Source: three-view drawing plus pictorial views. Frame: mm from the lowest corner of the part. A direction names the side the tool comes from. Round coordinates to 2 decimals unless told otherwise and drop trailing zeros. Order: outer loops, then holes, each group sorted by start corner. A loop starts at its lowest first (then second) coordinate and runs counter-clockwise, first axis right, second up. Notation, with made-up numbers: (-2.5, -20) -> (51.5, -20) arc R19 ccw to (51.5, -16) -> close; hole circle Ø10 at (89, -29). An arc over 180 degrees is marked (long way). Use a Markdown table: item, result.
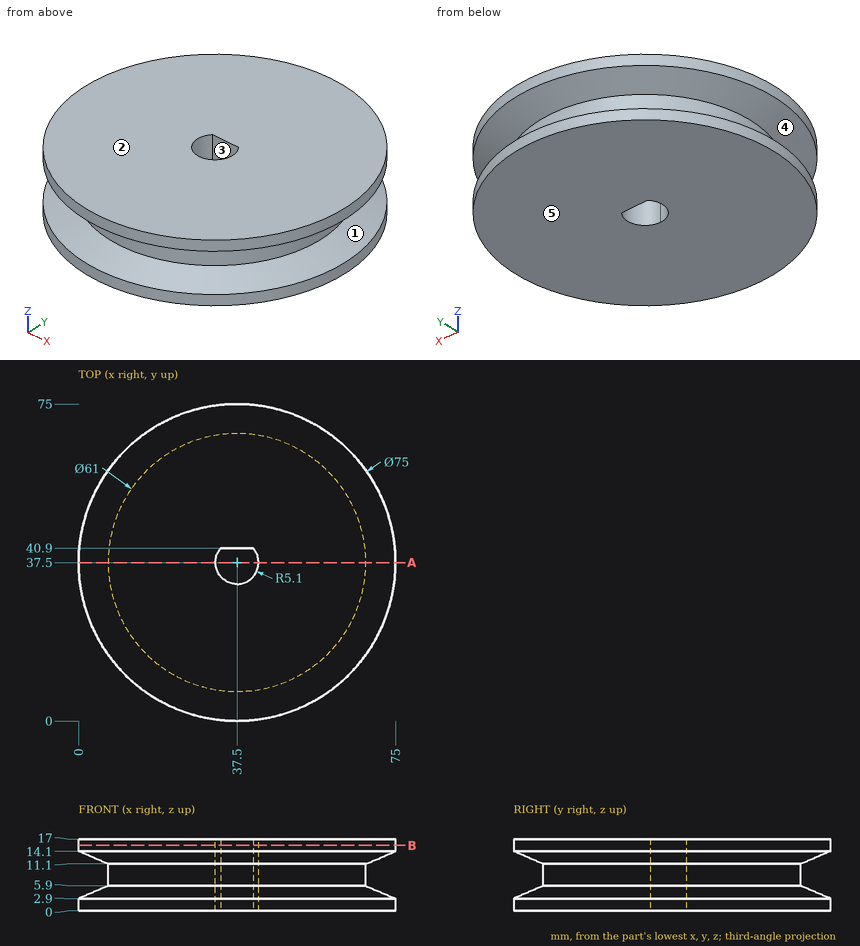
1) Cut plane B-B on z = 15.5. Return loops of the section in (x, y).
Results found:
| item | result |
|---|---|
| outline | circle Ø75 at (37.5, 37.5); hole (33.7, 40.9) arc R5.1 ccw (long way) to (41.3, 40.9) -> close |
2) Cut plane A-A on y = 37.5. Return loops of the section in (x, z), and give its area (3 significant figures).
Results found:
| item | result |
|---|---|
| outline | (0, 0) -> (32.4, 0) -> (32.4, 17) -> (0, 17) -> (0, 14.1) -> (7, 11.1) -> (7, 5.9) -> (0, 2.9) -> close; (42.6, 0) -> (75, 0) -> (75, 2.9) -> (68, 5.9) -> (68, 11.1) -> (75, 14.1) -> (75, 17) -> (42.6, 17) -> close |
| area | 987 mm² |
3) Line query: L1, parallel to Z at x = 4, y = 31.5; L2, parallel to Z at x = 60.5, y = 13; L3, parallel to X at y = 37, z = 9.25. Output: solid intervals per line, ascending. Write a range as [from, to].
Results found:
| item | result |
|---|---|
| L1 | z = [0, 4.39], [12.61, 17] |
| L2 | z = [0, 4.57], [12.43, 17] |
| L3 | x = [7, 32.42], [42.58, 68] |
4) Set-up query: the marked faces 4 and 5. Return all of +Z, -Z, +X, -X, +Y, -Y with unobstructed straight access to the full face (end or side cutting, diameter ignored); none if empty.
Results found:
| item | result |
|---|---|
| face 4 | none |
| face 5 | -Z, +X, -X, +Y, -Y |
5) Pull-direction query (Z, two-part tool) for the marked faces 1, 2 and 3; classes: +Z half, -Z half, draft (parallel to the pull), parting line (faces both ways), or undercut.
Results found:
| item | result |
|---|---|
| face 1 | undercut |
| face 2 | +Z half |
| face 3 | draft |
6) Pin query (flat end, axial travel): pin 1 Ø8.5 at (x, z) = (39.5, 8) entering from -Y; pin 2 Ø1.5 at (y, z) = (41, 4) entering from -X; pin 3 Ø1 at (x, z) = (48, 2.5) entering from +Y; pin 4 Ø5 at (x, y) = (47.5, 44.5) entering from -Z. Return the tip coordinate at first contact, or that it passes through.
Results found:
| item | result |
|---|---|
| pin 1 | stops at y = 2.04 |
| pin 2 | stops at x = 0.98 |
| pin 3 | stops at y = 73.64 |
| pin 4 | stops at z = 0 |
